The listing builds one solid part. Answer for the finished solid, in the listing's coordinates (mm). A direction names the side the tool comes from. Round coordinates to 2 decimals unless told otherwise and drop trailing zeros. Order: outer loops, then holes, each group sorted by start corner. A loop starts at its lowest first (then second) coordinate and runs counter-clockwise, first axis right, second up. Notation, with made-up numbers: (57.5, 30) - (72.5, 30) arc R22 ccw to (72.5, 46) - close; hole circle Ø1 at (-16.5, -13). An arc over 180 degrees is marked (long way). Write item = value, one per line.
from build123d import *

# Parameters (mm, degrees)
CUT_EXTRUDE1_DEPTH = 4.7625


with BuildPart() as part:
    # Sketch4 → Revolve1 (revolve)
    with BuildSketch(Plane(origin=(0, 0, 0), x_dir=(0, 0, -1), z_dir=(1, 0, 0)), mode=Mode.PRIVATE) as revolve1_sk:
        Polygon((-30.1625, 7.14375), (-35.798125, 7.14375), (-36.5125, 6.429375), (-36.5125, 0), (23.8125, 0), (23.8125, 4.500033333), (23.550033333, 4.7625), (-30.1625, 4.7625), align=None)
    revolve(revolve1_sk.sketch.rotate(Axis((0, 0, 36.5125), (0, 0, -1)), 90), axis=Axis((0, 0, 36.5125), (0, 0, -1)))

    # Sketch5 → Cut-Extrude1 (cut)
    with BuildSketch(Plane.XY.offset(36.5125)):
        Polygon((2.38125, 1.374815329), (0, 2.749630657), (-2.38125, 1.374815329), (-2.38125, -1.374815329), (0, -2.749630657), (2.38125, -1.374815329), align=None)
    extrude(amount=-CUT_EXTRUDE1_DEPTH, mode=Mode.SUBTRACT)

    # Cut-Extrude4 cone 1 section (on through the dimple's axis) → Cut-Extrude4 (revolve, cut)
    with BuildSketch(Plane(origin=(0, 0, 36.5125), x_dir=(0, -1, 0), z_dir=(1, 0, 0))):
        Polygon((0, 0), (2.749630657, 0), (0, 2.749630657), align=None)
    revolve(axis=Axis((0, 0, 36.5125), (0, 0, -1)), mode=Mode.SUBTRACT)

    # Sketch7 → Revolve2 (revolve)
    with BuildSketch(Plane(origin=(0, 0, 0), x_dir=(0, 0, -1), z_dir=(1, 0, 0)), mode=Mode.PRIVATE) as revolve2_sk:
        Polygon((23.8125, 3.9751), (35.454166667, 3.9751), (36.5125, 2.916766667), (36.5125, 0), (23.8125, 0), align=None)
    revolve(revolve2_sk.sketch.rotate(Axis((0, 0, -36.5125), (0, 0, 1)), 90), axis=Axis((0, 0, -36.5125), (0, 0, 1)))

    # Sketch10 → Cut-Revolve1 (revolve, cut)
    with BuildSketch(Plane(origin=(0, 0, 0), x_dir=(0, 0, -1), z_dir=(1, 0, 0)), mode=Mode.PRIVATE) as cut_revolve1_sk:
        with BuildLine():
            Line((24.6253, 3.1623), (26.6319, 3.1623))
            Line((26.6319, 3.1623), (28.2321, 4.7625))
            Line((28.2321, 4.7625), (23.8125, 4.7625))
            Line((23.8125, 4.7625), (23.8125, 3.9751))
            ThreePointArc((23.8125, 3.9751), (24.050563608, 3.400363608), (24.6253, 3.1623))
        make_face()
    revolve(cut_revolve1_sk.sketch.rotate(Axis((0, 0, -36.5125), (0, 0, 1)), 90), axis=Axis((0, 0, -36.5125), (0, 0, 1)), mode=Mode.SUBTRACT)


solid = part.part
Q1. Section B-B on z = 23 is taken. Determine the outline of the cut face in (x, y) (1 decimal), then the cut area to 3 significant figures.
Model answer:
outline = circle Ø9.5 at (0, 0)
area = 71.3 mm^2
Q2. Flat-ended cylindrical pins translate along their axes: P1, Ø2.5, axis at x = 1, y = 0, coming from the +Z side; P2, Ø4, axis at x = 1, z = 27, coming from the +Y side; P3, Ø4, axis at y = 1.5, z = 20, coming from the -X side. Find the tip coordinate at first contact, or state that the pin passes through.
Model answer:
P1 = 31.75
P2 = 4.76
P3 = -4.76
Q3. Determine the mould class of faces 4 (the face through (0, 0, -36.512)), 5 (the face through (-3, -1, -26)), 6 (the face through (-2.381, 0, 34)) for opening direction X: released by +X, released by -X, zero draft, split by the parting line, or undercut.
Model answer:
face_4 = zero draft
face_5 = split by the parting line
face_6 = undercut
Q4. For faces 1 (the face through (1.27, 2.23, 36.33)), 2 (the face through (3, 0, 36.512)), 3 (the face through (-3, 3, -23.812)), determine the directions among +Z, -Z, +X, -X, +Y, -Y from which every point of the face is accessible in a straight line to the end or side of a thin tool.
Model answer:
face_1 = +Z
face_2 = +Z, +X, -X, +Y, -Y
face_3 = -Z
Q5. Find the intervals of material crossed by line 1 (Z direction, x = -1, y = -0.75); line 2 (Z direction, x = 5.25, y = -0.5); line 3 (Y direction, x = 0, z = -20.5), in increasing order. Write a range as from..to.
Model answer:
line_1 = -36.51..31.75
line_2 = 30.16..36.51
line_3 = -4.76..4.76
